For this review, take the finished solid that the model builds, in its own axes (mm). A direction names the side the tool comes from. Give positions to 0.01 mm unless a question says otherwise; leave off trailing zeros. Loops run counter-clockwise (first coordinate to the right, second up) from the corner with the lowest first, then second, coordinate; pieces in that order, holes last. Notation, with made-up numbers: (52.5, 77.5) -> (62.5, 77.5) arc R22 ccw to (62.5, 112.5) -> close; hole circle Ø5 at (-10, -25). An arc over 180 degrees is marked (long way). Write each question's results on one line, items separated by ' | '. Start each with the question number.
Autodesk Inventor part; units mm, degrees
ref_plane "YZ Plane" through (0, 0, 0) normal (1, 0, 0) x (0, 1, 0)
ref_plane "XZ Plane" through (0, 0, 0) normal (0, 1, 0) x (-1, 0, 0)
ref_plane "XY Plane" through (0, 0, 0) normal (0, 0, 1) x (1, 0, 0)
sketch "スケッチ1" plane through (0, 0, 0) normal (0, 0, 1) x (1, 0, 0)
  circle A0 centre (0, 0) radius 12.5
  circle A1 centre (0, 0) radius 14
  circle A2 centre (0, 0) radius 18
  dimension "d0" = 25
  dimension "d1" = 28
  dimension "d2" = 36
extrude "押し出し1" add sketch "スケッチ1" along normal blind 1.5 contours A1 | A2
extrude "押し出し2" add sketch "スケッチ1" against normal blind 4 contours A1
properties part number "オイレスF　d25-D28-l12" material "アセタール樹脂、黒"
1. Draft analysis for pull direction Y (two halves, no side actions). For faces 1 (the cylindrical face through (12.932, -5.362, -1.972)), 2 (the cylindrical face through (11.923, -3.755, -1.288)), 3 (the flat face through (-5.3, 11.5, -4)), state which applies: released by +Y, released by -Y, zero draft, split by the parting line, or undercut.
2. Wall thickness on L1, parallel to Y at x = 0, z = -2.3; L2, parallel to Z at x = 14.5, y = 0.5; L3, parallel to X at y = -2, z = 0.7: over which ranges is each line inside the solid? List them lowest first.
3. We need section C-C (z = -1.9). Write out the cut boundary in (x, y).
4. We need section A-A (x = 0). Write out the cut boundary in (y, z).
5. Machinability: for faces 4 (the flat face through (9, -11, 0)), 5 (the cylindrical face through (-2.343, -17.847, 0.74)), which of the approach directions +Z, -Z, +X, -X, +Y, -Y give a long, thin tool a straight path to every point of the face, cutting with its end or side? Answer none if there is none.
6. For pin 1 Ø3 at (y, z) = (-6, -3) entering from +X, flat-tipped, find the tip position at first contact; note if it passes through.
7. We need section D-D (z = 0.6). Write out the cut boundary in (x, y).
Response:
1) face 1: split by the parting line | face 2: undercut | face 3: zero draft
2) L1: y = -14 to -12.5, 12.5 to 14 | L2: z = 0 to 1.5 | L3: x = -17.89 to -12.34, 12.34 to 17.89
3) outline: circle Ø28 at (0, 0); hole circle Ø25 at (0, 0)
4) outline: (-18, 0) -> (-14, 0) -> (-14, -4) -> (-12.5, -4) -> (-12.5, 1.5) -> (-18, 1.5) -> close; (12.5, -4) -> (14, -4) -> (14, 0) -> (18, 0) -> (18, 1.5) -> (12.5, 1.5) -> close
5) face 4: -Z | face 5: +Z, -Z
6) pin 1: stops at x = 13.26
7) outline: circle Ø36 at (0, 0); hole circle Ø25 at (0, 0)
